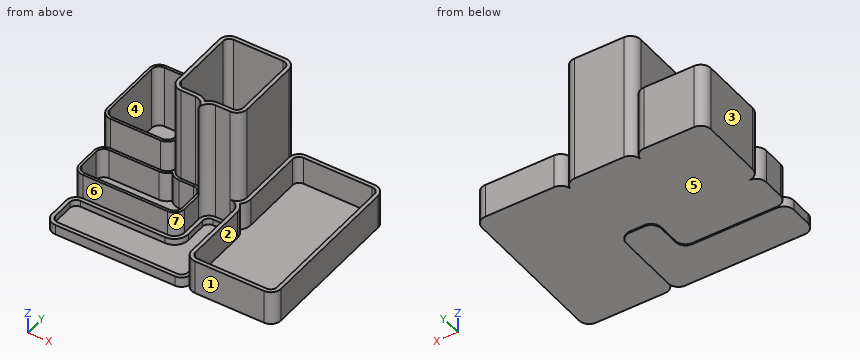
```python
from build123d import *

# Parameters (mm, degrees)
F1_DEPTH  = 3
F2_DEPTH  = 50
F3_DEPTH  = 100
F4_DEPTH  = 25
F5_DEPTH  = 25
F7_DEPTH  = 22
F8_DEPTH  = 2
F10_DEPTH = 97
F12_DEPTH = 50
F14_DEPTH = 24
F16_DEPTH = 5


with BuildPart() as f1:
    # F0 (on Top) → F1 (new body)
    with BuildSketch(Plane.XY):
        with BuildLine():
            Line((-82, -65), (11.900635, -65))
            ThreePointArc((11.900635, -65), (17.557489, -62.656854), (19.900635, -57))
            Line((19.900635, -57), (19.900635, -8))
            ThreePointArc((19.900635, -8), (17.557489, -2.343146), (11.900635, 0))
            Line((11.900635, 0), (0.535129, 0))
            ThreePointArc((0.535129, 0), (-5.121725, -2.343146), (-7.464871, -8))
            Line((-7.464871, -8), (-7.464871, -24.5))
            ThreePointArc((-7.464871, -24.5), (-9.808017, -30.156854), (-15.464871, -32.5))
            Line((-15.464871, -32.5), (-82, -32.5))
            ThreePointArc((-82, -32.5), (-87.656854, -34.843146), (-90, -40.5))
            Line((-90, -40.5), (-90, -57))
            ThreePointArc((-90, -57), (-87.656854, -62.656854), (-82, -65))
        make_face()
    extrude(amount=-F1_DEPTH)



with BuildPart() as f2:
    # F0 (on Top) → F2 (new body)
    with BuildSketch(Plane.XY):
        with BuildLine():
            ThreePointArc((-90, 8), (-87.656854, 2.343146), (-82, 0))
            Line((-82, 0), (-42.830377, 0))
            ThreePointArc((-42.830377, 0), (-37.173522, 2.343146), (-34.830377, 8))
            Line((-34.830377, 8), (-34.830377, 57))
            ThreePointArc((-34.830377, 57), (-37.173522, 62.656854), (-42.830377, 65))
            Line((-42.830377, 65), (-82, 65))
            ThreePointArc((-82, 65), (-87.656854, 62.656854), (-90, 57))
            Line((-90, 57), (-90, 8))
        make_face()
    extrude(amount=F2_DEPTH)


with BuildPart() as f1_1:
    add(f1.part)

    add(f2.part)  # F3 merges F2
    # F0 (on Top) → F3 (join)
    with BuildSketch(Plane.XY):
        with BuildLine():
            Line((0.535129, 0), (11.900635, 0))
            ThreePointArc((11.900635, 0), (17.557489, 2.343146), (19.900635, 8))
            Line((19.900635, 8), (19.900635, 57))
            ThreePointArc((19.900635, 57), (17.557489, 62.656854), (11.900635, 65))
            Line((11.900635, 65), (-26.830377, 65))
            ThreePointArc((-26.830377, 65), (-32.487231, 62.656854), (-34.830377, 57))
            Line((-34.830377, 57), (-34.830377, 8))
            ThreePointArc((-34.830377, 8), (-32.487231, 2.343146), (-26.830377, 0))
            Line((-26.830377, 0), (-15.464871, 0))
            ThreePointArc((-15.464871, 0), (-9.808017, -2.343146), (-7.464871, -8))
            ThreePointArc((-7.464871, -8), (-5.121725, -2.343146), (0.535129, 0))
        make_face()
    extrude(amount=F3_DEPTH)

    # F0 (on Top) → F4 (join)
    with BuildSketch(Plane.XY):
        with BuildLine():
            ThreePointArc((-90, -24.5), (-87.656854, -30.156854), (-82, -32.5))
            Line((-82, -32.5), (-15.464871, -32.5))
            ThreePointArc((-15.464871, -32.5), (-9.808017, -30.156854), (-7.464871, -24.5))
            Line((-7.464871, -24.5), (-7.464871, -8))
            ThreePointArc((-7.464871, -8), (-9.808017, -2.343146), (-15.464871, 0))
            Line((-15.464871, 0), (-26.830377, 0))
            ThreePointArc((-26.830377, 0), (-32.487231, 2.343146), (-34.830377, 8))
            ThreePointArc((-34.830377, 8), (-37.173522, 2.343146), (-42.830377, 0))
            Line((-42.830377, 0), (-82, 0))
            ThreePointArc((-82, 0), (-87.656854, -2.343146), (-90, -8))
            Line((-90, -8), (-90, -24.5))
        make_face()
    extrude(amount=F4_DEPTH)

    # F0 (on Top) → F5 (join)
    with BuildSketch(Plane.XY):
        with BuildLine():
            Line((19.900635, -8), (19.900635, -57))
            ThreePointArc((19.900635, -57), (22.243781, -62.656854), (27.900635, -65))
            Line((27.900635, -65), (82, -65))
            ThreePointArc((82, -65), (87.656854, -62.656854), (90, -57))
            Line((90, -57), (90, 57))
            ThreePointArc((90, 57), (87.656854, 62.656854), (82, 65))
            Line((82, 65), (27.900635, 65))
            ThreePointArc((27.900635, 65), (22.243781, 62.656854), (19.900635, 57))
            Line((19.900635, 57), (19.900635, 8))
            ThreePointArc((19.900635, 8), (17.557489, 2.343146), (11.900635, 0))
            ThreePointArc((11.900635, 0), (17.557489, -2.343146), (19.900635, -8))
        make_face()
    extrude(amount=F5_DEPTH)

    # F6 (on face) → F7 (cut)
    with BuildSketch(Plane.XY.offset(25)):
        with BuildLine():
            Line((22.900635, 57), (22.900635, 8))
            ThreePointArc((22.900635, 8), (22.001332, 3.643865), (19.450469, 0))
            ThreePointArc((19.450469, 0), (22.001332, -3.643865), (22.900635, -8))
            Line((22.900635, -8), (22.900635, -57))
            ThreePointArc((22.900635, -57), (24.365101, -60.535534), (27.900635, -62))
            Line((27.900635, -62), (82, -62))
            ThreePointArc((82, -62), (85.535534, -60.535534), (87, -57))
            Line((87, -57), (87, 57))
            ThreePointArc((87, 57), (85.535534, 60.535534), (82, 62))
            Line((82, 62), (27.900635, 62))
            ThreePointArc((27.900635, 62), (24.365101, 60.535534), (22.900635, 57))
        make_face()
    extrude(amount=-F7_DEPTH, mode=Mode.SUBTRACT)

    # F0 (on Top) → F8 (join)
    with BuildSketch(Plane.XY):
        with BuildLine():
            Line((19.900635, -8), (19.900635, -57))
            ThreePointArc((19.900635, -57), (22.243781, -62.656854), (27.900635, -65))
            Line((27.900635, -65), (82, -65))
            ThreePointArc((82, -65), (87.656854, -62.656854), (90, -57))
            Line((90, -57), (90, 57))
            ThreePointArc((90, 57), (87.656854, 62.656854), (82, 65))
            Line((82, 65), (27.900635, 65))
            ThreePointArc((27.900635, 65), (22.243781, 62.656854), (19.900635, 57))
            Line((19.900635, 57), (19.900635, 8))
            ThreePointArc((19.900635, 8), (17.557489, 2.343146), (11.900635, 0))
            ThreePointArc((11.900635, 0), (17.557489, -2.343146), (19.900635, -8))
        make_face()
        with BuildLine():
            Line((0.535129, 0), (11.900635, 0))
            ThreePointArc((11.900635, 0), (17.557489, 2.343146), (19.900635, 8))
            Line((19.900635, 8), (19.900635, 57))
            ThreePointArc((19.900635, 57), (17.557489, 62.656854), (11.900635, 65))
            Line((11.900635, 65), (-26.830377, 65))
            ThreePointArc((-26.830377, 65), (-32.487231, 62.656854), (-34.830377, 57))
            Line((-34.830377, 57), (-34.830377, 8))
            ThreePointArc((-34.830377, 8), (-32.487231, 2.343146), (-26.830377, 0))
            Line((-26.830377, 0), (-15.464871, 0))
            ThreePointArc((-15.464871, 0), (-9.808017, -2.343146), (-7.464871, -8))
            ThreePointArc((-7.464871, -8), (-5.121725, -2.343146), (0.535129, 0))
        make_face()
        with BuildLine():
            Line((-82, -65), (11.900635, -65))
            ThreePointArc((11.900635, -65), (17.557489, -62.656854), (19.900635, -57))
            Line((19.900635, -57), (19.900635, -8))
            ThreePointArc((19.900635, -8), (17.557489, -2.343146), (11.900635, 0))
            Line((11.900635, 0), (0.535129, 0))
            ThreePointArc((0.535129, 0), (-5.121725, -2.343146), (-7.464871, -8))
            Line((-7.464871, -8), (-7.464871, -24.5))
            ThreePointArc((-7.464871, -24.5), (-9.808017, -30.156854), (-15.464871, -32.5))
            Line((-15.464871, -32.5), (-82, -32.5))
            ThreePointArc((-82, -32.5), (-87.656854, -34.843146), (-90, -40.5))
            Line((-90, -40.5), (-90, -57))
            ThreePointArc((-90, -57), (-87.656854, -62.656854), (-82, -65))
        make_face()
        with BuildLine():
            ThreePointArc((-90, -24.5), (-87.656854, -30.156854), (-82, -32.5))
            Line((-82, -32.5), (-15.464871, -32.5))
            ThreePointArc((-15.464871, -32.5), (-9.808017, -30.156854), (-7.464871, -24.5))
            Line((-7.464871, -24.5), (-7.464871, -8))
            ThreePointArc((-7.464871, -8), (-9.808017, -2.343146), (-15.464871, 0))
            Line((-15.464871, 0), (-26.830377, 0))
            ThreePointArc((-26.830377, 0), (-32.487231, 2.343146), (-34.830377, 8))
            ThreePointArc((-34.830377, 8), (-37.173522, 2.343146), (-42.830377, 0))
            Line((-42.830377, 0), (-82, 0))
            ThreePointArc((-82, 0), (-87.656854, -2.343146), (-90, -8))
            Line((-90, -8), (-90, -24.5))
        make_face()
        with BuildLine():
            ThreePointArc((-90, 8), (-87.656854, 2.343146), (-82, 0))
            Line((-82, 0), (-42.830377, 0))
            ThreePointArc((-42.830377, 0), (-37.173522, 2.343146), (-34.830377, 8))
            Line((-34.830377, 8), (-34.830377, 57))
            ThreePointArc((-34.830377, 57), (-37.173522, 62.656854), (-42.830377, 65))
            Line((-42.830377, 65), (-82, 65))
            ThreePointArc((-82, 65), (-87.656854, 62.656854), (-90, 57))
            Line((-90, 57), (-90, 8))
        make_face()
    extrude(amount=-F8_DEPTH)

    # F9 (on face) → F10 (cut)
    with BuildSketch(Plane.XY.offset(100)):
        with BuildLine():
            Line((-26.830377, 3), (-15.464871, 3))
            ThreePointArc((-15.464871, 3), (-11.108736, 2.100697), (-7.464871, -0.450166))
            ThreePointArc((-7.464871, -0.450166), (-3.821006, 2.100697), (0.535129, 3))
            Line((0.535129, 3), (11.900635, 3))
            ThreePointArc((11.900635, 3), (15.436169, 4.464466), (16.900635, 8))
            Line((16.900635, 8), (16.900635, 57))
            ThreePointArc((16.900635, 57), (15.436169, 60.535534), (11.900635, 62))
            Line((11.900635, 62), (-26.830377, 62))
            ThreePointArc((-26.830377, 62), (-30.36591, 60.535534), (-31.830377, 57))
            Line((-31.830377, 57), (-31.830377, 8))
            ThreePointArc((-31.830377, 8), (-30.36591, 4.464466), (-26.830377, 3))
        make_face()
    extrude(amount=-F10_DEPTH, mode=Mode.SUBTRACT)

    # F11 (on face) → F12 (cut)
    with BuildSketch(Plane.XY.offset(50)):
        with BuildLine():
            Line((-88, 57), (-88, 8))
            ThreePointArc((-88, 8), (-86.242641, 3.757359), (-82, 2))
            Line((-82, 2), (-42.830377, 2))
            ThreePointArc((-42.830377, 2), (-38.587736, 3.757359), (-36.830377, 8))
            Line((-36.830377, 8), (-36.830377, 57))
            ThreePointArc((-36.830377, 57), (-38.587736, 61.242641), (-42.830377, 63))
            Line((-42.830377, 63), (-82, 63))
            ThreePointArc((-82, 63), (-86.242641, 61.242641), (-88, 57))
        make_face()
    extrude(amount=-F12_DEPTH, mode=Mode.SUBTRACT)

    # F13 (on face) → F14 (cut)
    with BuildSketch(Plane.XY.offset(25)):
        with BuildLine():
            Line((-88, -8), (-88, -24.5))
            ThreePointArc((-88, -24.5), (-86.242641, -28.742641), (-82, -30.5))
            Line((-82, -30.5), (-15.464871, -30.5))
            ThreePointArc((-15.464871, -30.5), (-11.22223, -28.742641), (-9.464871, -24.5))
            Line((-9.464871, -24.5), (-9.464871, -8))
            ThreePointArc((-9.464871, -8), (-11.22223, -3.757359), (-15.464871, -2))
            Line((-15.464871, -2), (-26.830377, -2))
            ThreePointArc((-26.830377, -2), (-31.302512, -0.944272), (-34.830377, 2))
            ThreePointArc((-34.830377, 2), (-38.358241, -0.944272), (-42.830377, -2))
            Line((-42.830377, -2), (-82, -2))
            ThreePointArc((-82, -2), (-86.242641, -3.757359), (-88, -8))
        make_face()
    extrude(amount=-F14_DEPTH, mode=Mode.SUBTRACT)

    # F15 (on face) → F16 (join)
    with BuildSketch(Plane.XY):
        with BuildLine():
            ThreePointArc((-90, -57), (-87.656854, -62.656854), (-82, -65))
            Line((-82, -65), (11.900635, -65))
            ThreePointArc((11.900635, -65), (17.557489, -62.656854), (19.900635, -57))
            Line((19.900635, -57), (19.900635, -8))
            ThreePointArc((19.900635, -8), (17.557489, -2.343146), (11.900635, 0))
            Line((11.900635, 0), (0.535129, 0))
            ThreePointArc((0.535129, 0), (-5.121725, -2.343146), (-7.464871, -8))
            Line((-7.464871, -8), (-7.464871, -24.5))
            ThreePointArc((-7.464871, -24.5), (-9.808017, -30.156854), (-15.464871, -32.5))
            Line((-15.464871, -32.5), (-82, -32.5))
            ThreePointArc((-82, -32.5), (-87.656854, -34.843146), (-90, -40.5))
            Line((-90, -40.5), (-90, -57))
        make_face()
        with BuildLine():
            ThreePointArc((16.900635, -57), (15.436169, -60.535534), (11.900635, -62))
            Line((11.900635, -62), (-82, -62))
            ThreePointArc((-82, -62), (-85.535534, -60.535534), (-87, -57))
            Line((-87, -57), (-87, -40.5))
            ThreePointArc((-87, -40.5), (-85.535534, -36.964466), (-82, -35.5))
            Line((-82, -35.5), (-15.464871, -35.5))
            ThreePointArc((-15.464871, -35.5), (-7.686696, -32.278175), (-4.464871, -24.5))
            Line((-4.464871, -24.5), (-4.464871, -8))
            ThreePointArc((-4.464871, -8), (-3.000405, -4.464466), (0.535129, -3))
            Line((0.535129, -3), (11.900635, -3))
            ThreePointArc((11.900635, -3), (15.436169, -4.464466), (16.900635, -8))
            Line((16.900635, -8), (16.900635, -57))
        make_face(mode=Mode.SUBTRACT)
    extrude(amount=F16_DEPTH)


solid = f1_1.part
```
Work out the finished part from the listing and answer in its coordinate system (mm). Face numbers are marked on the shaded views. A direction names the side the tool comes from. Round coordinates to 2 decimals unless told otherwise and drop trailing zeros. Loops run counter-clockwise (first coordinate to the right, second up) from the corner with the lowest first, then second, coordinate; pieces in that order, holes last. Notation, with made-up numbers: (62.25, 87.25) -> (96.25, 87.25) arc R22 cw to (96.25, 110.25) -> close; hole circle Ø2 at (-6.75, 81). An arc over 180 degrees is marked (long way). Write each question's results on one line, items separated by ' | '. Start each with the question number.
1. Section D-D (z = 44) is taken. State how many separate pieces and enclosed holes the cut face has, plus the area to 3 significant figures.
2. Section A-A (z = 61.5) is taken. Determine the outline of the cut face in (x, y), plus the area to 3 significant figures.
3. Section C-C (y = -14) is taken. Determine the outline of the cut face in (x, z).
4. Find the intervals of material crossed by probe 1 along Y at (x, z) = (-78, 18.5); probe 2 along Y at (x, z) = (-44.5, 2); probe 3 along Y at (x, z) = (8.5, 15), in increasing order. Write a range as from..to.
5. For a pull along X with two mould halves and no side action, classify the marked faces 1, 2 and 3 as +X half, -X half, draft (parallel to the pull), parting line (faces both ways), or undercut.
6. A tool of negligible diameter and unlimited length cuts with its end or side. For the marked faces 4, 5, 6 and 7, from which of +Z, -Z, +X, -X, +Y, -Y can it reach the whole face along a straight path? Write none if from no direction.
7. Given pin 1 Ø4 at (y, z) = (31, 42) entering from +X; pin 2 Ø8 at (x, y) = (4, 15.5) entering from -Z; pin 3 Ø16.5 at (x, y) = (-56, 35.5) entering from +Z, each flat-ended and moving along its own axis, determine where each tip first touches the part or whether it passes through.
8. Section B-B (x = 62) is taken. Determine the outline of the cut face in (y, z), plus the area to 3 significant figures.
Evaluation:
1) separate pieces: 1 | enclosed holes: 2 | area: 1,100 mm2
2) outline: (-34.83, 8) arc R8 ccw to (-26.83, 0) -> (-15.46, 0) arc R8 cw to (-7.46, -8) arc R8 cw to (0.54, 0) -> (11.9, 0) arc R8 ccw to (19.9, 8) -> (19.9, 57) arc R8 ccw to (11.9, 65) -> (-26.83, 65) arc R8 ccw to (-34.83, 57) -> close; hole (-31.83, 8) arc R5 ccw to (-26.83, 3) -> (-15.46, 3) arc R11 cw to (-7.46, -0.45) arc R11 cw to (0.54, 3) -> (11.9, 3) arc R5 ccw to (16.9, 8) -> (16.9, 57) arc R5 ccw to (11.9, 62) -> (-26.83, 62) arc R5 ccw to (-31.83, 57) -> close | area: 659 mm2
3) outline: (-90, -2) -> (-7.46, -2) -> (-7.46, -3) -> (19.9, -3) -> (19.9, -2) -> (90, -2) -> (90, 25) -> (87, 25) -> (87, 3) -> (22.9, 3) -> (22.9, 25) -> (19.9, 25) -> (19.9, 5) -> (16.9, 5) -> (16.9, 0) -> (-4.46, 0) -> (-4.46, 5) -> (-7.46, 5) -> (-7.46, 25) -> (-9.46, 25) -> (-9.46, 1) -> (-88, 1) -> (-88, 25) -> (-90, 25) -> close
4) probe 1: y = -32.5..-30.5, -2..2, 63..65 | probe 2: y = -65..-62, -35.5..-30.5, -2..2, 63..65 | probe 3: y = 0..3, 62..65
5) face 1: draft | face 2: undercut | face 3: -X half
6) face 4: +Z | face 5: -Z, +Y | face 6: +Z, -X, -Y | face 7: +Z, -Y
7) pin 1: stops at x = 19.9 | pin 2: stops at z = -2 | pin 3: stops at z = 0
8) outline: (-65, -2) -> (65, -2) -> (65, 25) -> (62, 25) -> (62, 3) -> (-62, 3) -> (-62, 25) -> (-65, 25) -> close | area: 782 mm2
